```python
from build123d import *

# Parameters (mm, degrees)
F0_W      = 500
F0_H      = 500
F1_DEPTH  = 950
F2_T      = -19
F3_W      = 400
F3_H      = 900
F4_DEPTH  = 25
F5_R      = 10
F7_W      = 461.7021232843
F7_H      = 462.5295698643
F8_DEPTH  = 19
F10_W     = 460.7798308134
F10_H     = 461.6745561361
F11_DEPTH = 19


with BuildPart() as f1:
    # F0 (on Top) → F1 (new body)
    with BuildSketch(Plane.XY):
        Rectangle(F0_W, F0_H)
    extrude(amount=F1_DEPTH)

    # F2
    f2_openings = [f1.faces().sort_by_distance(p)[0] for p in [
        (0, 0, 0),
    ]]
    offset(amount=F2_T, openings=f2_openings)

    # F3 (on face) → F4 (cut)
    with BuildSketch(Plane.YZ.offset(250)):
        with Locations((0, 450)):
            Rectangle(F3_W, F3_H)
    extrude(amount=-F4_DEPTH, mode=Mode.SUBTRACT)

    # F5
    f5_edges = [f1.edges().sort_by_distance(p)[0] for p in [
        (240.5, 200, 900),
        (240.5, -200, 900),
    ]]
    fillet(f5_edges, radius=F5_R)

    # F7 (on offset) → F8 (join)
    with BuildSketch(Plane.XY.offset(100)):
        with Locations((-0.2068504691, 0.2068579197)):
            Rectangle(F7_W, F7_H)
    extrude(amount=F8_DEPTH)

    # F10 (on offset) → F11 (join)
    with BuildSketch(Plane.XY.offset(469)):
        with Locations((0.1056715846, -0.2236738801)):
            Rectangle(F10_W, F10_H)
    extrude(amount=F11_DEPTH)


solid = f1.part
```
The listing builds one solid part. Answer for the finished solid, in the listing's coordinates (mm). A direction names the side the tool comes from. Coordinates: 2 decimals unless noted, no trailing zeros. Write each loop counter-clockwise with the first axis right and the second up, starting at its lowest first coordinate (ties: lowest second). Pieces come first, ordered by that corner, then holes. Notation, with made-up numbers: (55.5, 39) - (84.5, 39) arc R19 cw to (84.5, 53) - close; hole circle Ø7 at (15, 7.5). An arc over 180 degrees is marked (long way). Return JSON: item names as keys, results as strings. Group by question number.
Q1. The part is cut by section A-A on y = 81. Write down the section's boundary in (x, z).
Q2. The part is cut by section C-C on z = 254. Write down the section's boundary in (x, y).
Q3. Which of the six approach directions +Z, -Z, +X, -X, +Y, -Y give full straight-line access (tool end or side, diameter ignored) to faces 5 (the flat face through (-230.284, -3, 478)), 6 (the flat face through (241, -3, 900))?
Q4. The part is cut by section B-B on x = -147.5. Write down the section's boundary in (y, z).
Q5. For a pull along Z with two mould halves and no side action, classify faces 1 (the flat face through (-3, 3, 488)), 2 (the flat face through (241, 200, 439)), 3 (the flat face through (-3, 4, 950)), 4 (the flat face through (-3, 3, 931)) as +Z half, -Z half, draft (parallel to the pull), parting line (faces both ways), or undercut.
Q6. Find the intervals of material crossed by line 1 along Z through (x, y) = (195, 193); line 2 along X through (y, z) = (224, 484); line 3 along Y through (x, z) = (-179.5, 486), in increasing order. Write a range as [from, to].
Q7. Flat-ended cylindrical pins translate along their axes: pin 1 Ø15 at (y, z) = (-53, 483) entering from +X; pin 2 Ø3 at (y, z) = (59.5, 396) entering from +X; pin 3 Ø5.5 at (x, y) = (237, 92) entering from -Z. Find the tip coordinate at first contact, or state that the pin passes through.
Evaluation:
{
 "1": {"outline": "(-250, 0) - (-231, 0) - (-231, 100) - (230.64, 100) - (230.64, 119) - (-231, 119) - (-231, 931) - (231, 931) - (231, 900) - (250, 900) - (250, 950) - (-250, 950) - close; (-230.28, 469) - (230.5, 469) - (230.5, 488) - (-230.28, 488) - close"},
 "2": {"outline": "(-250, -250) - (250, -250) - (250, -200) - (231, -200) - (231, -231) - (-231, -231) - (-231, 231) - (231, 231) - (231, 200) - (250, 200) - (250, 250) - (-250, 250) - close"},
 "3": {"face 5": "none", "face 6": "-Z, +X"},
 "4": {"outline": "(-250, 0) - (-231, 0) - (-231, 100) - (231, 100) - (231, 0) - (250, 0) - (250, 950) - (-250, 950) - close; hole (-231, 119) - (231, 119) - (231, 931) - (-231, 931) - (-231, 488) - (230.61, 488) - (230.61, 469) - (-231, 469) - close"},
 "5": {"face 1": "undercut", "face 2": "draft", "face 3": "+Z half", "face 4": "undercut"},
 "6": {"line 1": "z = [100, 119], [469, 488], [931, 950]", "line 2": "x = [-250, -231], [-230.28, 230.5], [231, 250]", "line 3": "y = [-250, 230.61], [231, 250]"},
 "7": {"pin 1": "stops at x = 230.5", "pin 2": "stops at x = -231", "pin 3": "stops at z = 900"}
}
